Geometry: final body of the model. Coordinates: model frame, mm. Face numbers are marked on the shaded views. A direction names the side the tool comes from. Round coordinates to 2 decimals unless told otherwise and drop trailing zeros. Write each loop counter-clockwise with the first axis right and the second up, starting at its lowest first coordinate (ties: lowest second). Pieces come first, ordered by that corner, then holes. Notation, with made-up numbers: (8, 74) -> (23, 74) arc R26 ccw to (23, 108) -> close; hole circle Ø3 at (58.25, -2). An arc over 180 degrees is marked (long way). Use one line per item in the form item = value. Start each with the question number.
1. Pin query (flat end, axial travel): pin 1 Ø4.5 at (x, z) = (-25.5, -3) entering from -Y; pin 2 Ø1.5 at (y, z) = (-9.5, 12.5) entering from -X (3 decimals); pin 3 Ø2 at (x, z) = (4.5, -4.5) entering from +Y. Return the tip coordinate at first contact, or that it passes through.
2. Cut plane B-B, the plane x = -5. Return the cut outline in (y, z) (3 decimals).
3. Line query: L1, parallel to X at y = -14.5, z = 15 (3 decimals); L2, parallel to Y at x = 0.5, z = 14.5; L3, parallel to Y at x = 21, z = -17. Output: solid intervals per line, ascending.
4. Reachability of the marked faces 1, 2, 3, 4 and 5 from +Z, -Z, +X, -X, +Y, -Y: full face, straight path, thin tool, end or side. Return the list, or none.
5. Cut plane D-D, the plane x = 3.5. Return the cut outline in (y, z) (1 decimal), plus the area to 3 significant figures.
6. Cut plane A-A, the plane z = 1. Return the cut outline in (x, y) (1 decimal), plus the area to 3 significant figures.
7. Cut plane C-C, the plane y = -12. Return the cut outline in (x, z) (3 decimals).
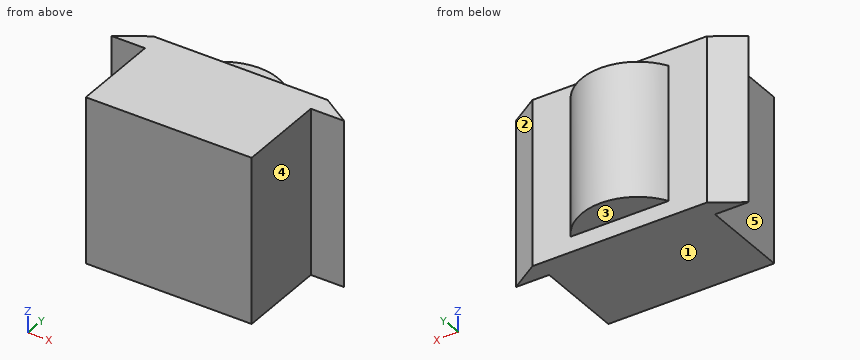
```python
from build123d import *

# Parameters (mm, degrees)
BOSS_EXTRUDE1_DEPTH = 22.225
SKETCH2_W           = 26.27393882
SKETCH2_H           = 4.154599903
CUT_EXTRUDE1_DEPTH  = 44.45


with BuildPart() as part:
    # Sketch1 → Boss-Extrude1 (new body, symmetric)
    with BuildSketch(Plane.XY):
        with BuildLine():
            Line((-23.369890455, 7.407032893), (-13.13696941, 7.407032893))
            ThreePointArc((-13.13696941, 7.407032893), (0, 15.08125), (13.13696941, 7.407032893))
            Line((13.13696941, 7.407032893), (23.369890455, 7.407032893))
            Line((23.369890455, 7.407032893), (31.15985394, 2.38125))
            Line((31.15985394, 2.38125), (22.225, 2.38125))
            Line((22.225, 2.38125), (22.225, -21.51875))
            Line((22.225, -21.51875), (-22.225, -21.51875))
            Line((-22.225, -21.51875), (-22.225, 2.38125))
            Line((-22.225, 2.38125), (-31.15985394, 2.38125))
            Line((-31.15985394, 2.38125), (-23.369890455, 7.407032893))
        make_face()
    extrude(amount=BOSS_EXTRUDE1_DEPTH, both=True)

    # Sketch2 → Cut-Extrude1 (cut)
    with BuildSketch(Plane(origin=(0, 7.407032893, 0), x_dir=(1, 0, 0), z_dir=(0, 1, 0))):
        with Locations((0, 20.147700048)):
            Rectangle(SKETCH2_W, SKETCH2_H)
        with Locations((0, -20.147700048)):
            Rectangle(SKETCH2_W, SKETCH2_H)
    extrude(amount=CUT_EXTRUDE1_DEPTH, mode=Mode.SUBTRACT)


solid = part.part
```
Outcome:
q1.pin_1 = 2.38
q1.pin_2 = -22.225
q1.pin_3 = 14.67
q2.outline = (-21.519, -22.225) -> (7.407, -22.225) -> (7.407, -18.07) -> (14.228, -18.07) -> (14.228, 18.07) -> (7.407, 18.07) -> (7.407, 22.225) -> (-21.519, 22.225) -> close
q3.L1 = -22.225 to 22.225
q3.L2 = -21.52 to 15.07
q3.L3 = -21.52 to 7.41
q4.face_1 = -Z, +X, -X, +Y, -Y
q4.face_2 = +Z, -Z, +X, +Y
q4.face_3 = -Z, +X, -X, +Y
q4.face_4 = +Z, -Z, +X, -Y
q4.face_5 = +Z, -Z, -X, -Y
q5.outline = (-21.5, -22.2) -> (7.4, -22.2) -> (7.4, -18.1) -> (14.7, -18.1) -> (14.7, 18.1) -> (7.4, 18.1) -> (7.4, 22.2) -> (-21.5, 22.2) -> close
q5.area = 1,550 mm^2
q6.outline = (-31.2, 2.4) -> (-22.2, 2.4) -> (-22.2, -21.5) -> (22.2, -21.5) -> (22.2, 2.4) -> (31.2, 2.4) -> (23.4, 7.4) -> (13.1, 7.4) arc R15.1 ccw to (-13.1, 7.4) -> (-23.4, 7.4) -> close
q6.area = 1,480 mm^2
q7.outline = (-22.225, -22.225) -> (22.225, -22.225) -> (22.225, 22.225) -> (-22.225, 22.225) -> close
